```python
from build123d import *

# Parameters (mm, degrees)
F0_R     = 40
F1_DEPTH = 2
F2_R     = 38.5
F3_DEPTH = 5
F7_R     = 15
F4_R     = 40
F9_T     = -2


with BuildPart() as f1:
    # F0 (on Top) → F1 (new body)
    with BuildSketch(Plane.XY):
        Circle(F0_R)
    extrude(amount=F1_DEPTH)

    # F2 (on face) → F3 (join)
    with BuildSketch(Plane.XY.offset(2)):
        Circle(F2_R)
    extrude(amount=F3_DEPTH)

    # F7 (on plane+point) → F8 section 0
    with BuildSketch(Plane.XY.offset(-130.1585063338)):
        Circle(F7_R)
    # F4 (on face) → F8 section 1
    with BuildSketch(Plane(origin=(0, 0, 0), x_dir=(1, 0, 0), z_dir=(0, 0, -1))):
        Circle(F4_R)
    loft()

    # F9
    f9_openings = [f1.faces().sort_by_distance(p)[0] for p in [
        (0, 0, -130.158506),
    ]]
    offset(amount=F9_T, openings=f9_openings, kind=Kind.INTERSECTION)


solid = f1.part
```
Verification items for the finished model (mm, model axes). A direction names the side the tool comes from. Coordinates: 2 decimals unless noted, no trailing zeros. Write each loop counter-clockwise with the first axis right and the second up, starting at its lowest first coordinate (ties: lowest second). Pieces come first, ordered by that corner, then holes. Notation, with made-up numbers: M 13.25,67.5 L 43.25,67.5 A6 cw 43.25,73.5 Z; hole C 14,1 d1. An arc over 180 degrees is marked long. Answer as a JSON object with one key per item and string values. Group by question number.
(1) Tool access check on faces 1 (the face through (-20, 31, 0)), 2 (the face through (-5.999, -27.017, -64.168)), 3 (the face through (-21, 33, 2)). Record the directions out of +Z, -Z, +X, -X, +Y, -Y that give a thin tool (end or side, any length) a straight path to the whole face; none if there is none.
(2) Material ranges on line 1 (Y direction, x = 0, z = 2.2); line 2 (Y direction, x = 0, z = 1.9); line 3 (Z direction, x = -2.5, y = -10), recorded low to high.
(3) Cross-section at C-C, the plane z = -17. Record the cut outline in (x, y), and give its area (3 significant figures).
(4) Cross-section at B-B, the plane z = -96.5. Record the cut outline in (x, y), and give its area (3 significant figures).
(5) Cross-section at A-A, the plane x = 0. Record the cut outline in (y, z).
(6) Release check for a two-part mould opening along Y. For faces 4 (the face through (-7.912, -35.632, 2.465)), 5 (the face through (-13.4, 0.1, -130.159)), 6 (the face through (-30.55, -23.43, 4.46)) record: +Y half, -Y half, draft (parallel to the pull), parting line (faces both ways), or undercut.
(7) Gauge pin test, flat end, axial feed: pin 1 (10 mm diameter, centred on y = 4.5, z = -26.5, fed in from -X). Record the tip position at first contact, or that the pin passes through.
Reply:
{
 "1": {"face 1": "none", "face 2": "-Z", "face 3": "+Z"},
 "2": {"line 1": "-38.5 to -36.5, 36.5 to 38.5", "line 2": "-40 to -36.5, 36.5 to 40", "line 3": "5 to 7"},
 "3": {"outline": "C 0,0 d73.47; hole C 0,0 d69.4", "area": "457 mm²"},
 "4": {"outline": "C 0,0 d42.93; hole C 0,0 d38.86", "area": "262 mm²"},
 "5": {"outline": "M -40,0 L -15,-130.16 L -12.96,-130.16 L -37.96,0 L -36.5,0 L -36.5,5 L 36.5,5 L 36.5,0 L 37.96,0 L 12.96,-130.16 L 15,-130.16 L 40,0 L 40,2 L 38.5,2 L 38.5,7 L -38.5,7 L -38.5,2 L -40,2 Z"},
 "6": {"face 4": "undercut", "face 5": "draft", "face 6": "parting line"},
 "7": {"pin 1": "x = -35.7"}
}
